```python
from build123d import *

# Parameters (mm, degrees)
SKETCH_1_R          = 1.6
EXTRUDE_1_DEPTH     = 2
SKETCH_2_R          = 2.5
EXTRUDE_2_DEPTH     = 30
FILLET_1_R          = 0.5
SKETCH_3_R          = 0.75
CUT_EXTRUDE_1_DEPTH = 35.165040612
SKETCH_4_W          = 5.098076211
SKETCH_4_H          = 16
CUT_EXTRUDE_2_DEPTH = 34.841542518


with BuildPart() as part:
    # 草图1 → 凸台-拉伸1 (new body)
    with BuildSketch(Plane(origin=(0, 0, 0), x_dir=(1, 0, 0), z_dir=(0, 1, 0))):
        with BuildLine():
            Line((3, 0), (12.5, 0))
            Line((12.5, 0), (12.5, -30))
            Line((12.5, -30), (3, -30))
            ThreePointArc((3, -30), (0.878679656, -29.121320344), (0, -27))
            Line((0, -27), (0, -3))
            ThreePointArc((0, -3), (0.878679656, -0.878679656), (3, 0))
        make_face()
        with Locations(Location((4.5, -5, 0), (0, 0, 270))):
            Circle(SKETCH_1_R, mode=Mode.SUBTRACT)
        with Locations(Location((4.5, -25, 0), (0, 0, 270))):
            Circle(SKETCH_1_R, mode=Mode.SUBTRACT)
    extrude(amount=EXTRUDE_1_DEPTH)

    # 草图2 → 凸台-拉伸2 (add)
    with BuildSketch(Plane.XY.offset(30)):
        with Locations((12.5, 4)):
            Circle(SKETCH_2_R)
    extrude(amount=-EXTRUDE_2_DEPTH)

    # 圆角1
    fillet_1_edges = [part.edges().sort_by_distance(p)[0] for p in [
        (12.5, 1.5, 15),
        (11, 2, 15),
        (12.5, 0, 15),
    ]]
    fillet(fillet_1_edges, radius=FILLET_1_R)

    # 草图3 → 切除-拉伸1 (cut, through all)
    with BuildSketch(Plane.XY.offset(30)):
        with Locations((12.5, 4)):
            Circle(SKETCH_3_R)
    extrude(amount=-CUT_EXTRUDE_1_DEPTH, mode=Mode.SUBTRACT)

    # 草图4 → 切除-拉伸2 (cut, through all)
    with BuildSketch(Plane(origin=(0, 2, 0), x_dir=(1, 0, 0), z_dir=(0, 1, 0))):
        with Locations((12.450961895, -15)):
            Rectangle(SKETCH_4_W, SKETCH_4_H)
    extrude(amount=CUT_EXTRUDE_2_DEPTH, mode=Mode.SUBTRACT)


solid = part.part
```
Source: CAD feature listing. Evaluate the final solid. Frame: model axes, mm. A direction names the side the tool comes from. Give positions to 0.01 mm unless a question says otherwise; leave off trailing zeros. Loops run counter-clockwise (first coordinate to the right, second up) from the corner with the lowest first, then second, coordinate; pieces in that order, holes last. Notation, with made-up numbers: (-23, -11) -> (7, -11) arc R16 ccw to (7, -5) -> close; hole circle Ø7 at (29, -20). An arc over 180 degrees is marked (long way). Use a Markdown table: item, result. Add a question column.
(1) Section query D-D (z = 18.5). Output: boundary loops of the cut face in (x, y), then the cut area to 3 significant figures.
(2) Section query B-B (z = 5). Output: boundary loops of the cut face in (x, y).
(3) Section query C-C (y = 4). Output: boundary loops of the cut face in (x, z).
(4) First-contact query: pin 1 Ø1 at (x, y) = (13, 2.5) entering from -Z; pin 2 Ø3 at (x, z) = (3, 24) entering from +Y; pin 3 Ø1.2 at (x, y) = (12.5, 4) entering from -Z. Flat tips, straight axial feed; report the tip coordinate or a pass-through.
(5) Section query A-A (y = 5.5). Output: boundary loops of the cut face in (x, z).
(6) Pull-direction query (X, two-part tool) for faces 1 (the face through (13.5, 1.71, 15.21)), 2 (the face through (11.75, 4.03, 3.55)), 3 (the face through (13, 5, 7)); classes: +X half, -X half, draft (parallel to the pull), parting line (faces both ways), or undercut.
(7) Access query for faces 4 (the face through (7, 2, 15)), 5 (the face through (0.86, 0.99, 0.9)), 6 (the face through (13, 5, 23)). Directions: +Z, -Z, +X, -X, +Y, -Y. A direction counts if a zero-diameter tool reaches every point of the face in a straight line with its end or side. Return the directions, or none.
(8) Ray query, line 1 (Z direction, x = 12, y = 5.5); line 2 (X direction, y = 0.95, z = 5); line 3 (Y direction, x = 11, z = 22). Return the intervals inside material, ascending.
Checked values:
| question | item | result |
|---|---|---|
| 1 | outline | (0, 0) -> (12, 0) arc R0.5 ccw to (12.5, 0.5) -> (12.5, 1.04) arc R0.5 cw to (12.92, 1.53) arc R2.5 ccw to (14, 2) -> (0, 2) -> close |
| 1 | area | 25.5 mm^2 |
| 2 | outline | (0, 0) -> (2.9, 0) -> (2.9, 2) -> (0, 2) -> close; (6.1, 0) -> (12, 0) arc R0.5 ccw to (12.5, 0.5) -> (12.5, 1.04) arc R0.5 cw to (12.92, 1.53) arc R2.5 ccw (long way) to (10.33, 2.75) arc R0.5 cw to (9.9, 2) -> (6.1, 2) -> close; hole circle Ø1.5 at (12.5, 4) |
| 3 | outline | (10, 0) -> (11.75, 0) -> (11.75, 7) -> (10, 7) -> close; (10, 23) -> (11.75, 23) -> (11.75, 30) -> (10, 30) -> close; (13.25, 0) -> (15, 0) -> (15, 7) -> (13.25, 7) -> close; (13.25, 23) -> (15, 23) -> (15, 30) -> (13.25, 30) -> close |
| 4 | pin 1 | z = 0 |
| 4 | pin 2 | y = 2 |
| 4 | pin 3 | through |
| 5 | outline | (10.5, 0) -> (14.5, 0) -> (14.5, 7) -> (10.5, 7) -> close; (10.5, 23) -> (14.5, 23) -> (14.5, 30) -> (10.5, 30) -> close |
| 6 | face 1 | parting line |
| 6 | face 2 | undercut |
| 6 | face 3 | draft |
| 7 | face 4 | -X, +Y |
| 7 | face 5 | -Z, -X, +Y, -Y |
| 7 | face 6 | +X, -X, +Y |
| 8 | line 1 | 0 to 7, 23 to 30 |
| 8 | line 2 | 0 to 2.9, 6.1 to 12.5 |
| 8 | line 3 | 0 to 2 |
